CAD build for the part. Positions are in the model's coordinates, mm. Coordinates: 2 decimals unless noted, no trailing zeros. Write each loop counter-clockwise with the first axis right and the second up, starting at its lowest first coordinate (ties: lowest second). Pieces come first, ordered by that corner, then holes.
Autodesk Inventor part; units mm, degrees
ref_plane "Start Plane" through (0, 0, 0) normal (1, 0, 0) x (0, 1, 0)
ref_plane "XZ Plane" through (0, 0, 0) normal (0, 1, 0) x (-1, 0, 0)
ref_plane "XY Plane" through (0, 0, 0) normal (0, 0, 1) x (1, 0, 0)
sketch "Main Sketch" plane through (0, 0, 0) normal (0, 0, 1) x (1, 0, 0)
  line L0 (0, 0) -> (914.4, 0)
  line L1 (0, 0) -> (0, 6.35)
  line L2 (914.4, 6.35) -> (914.4, 0)
  line L3 (0, 6.35) -> (914.4, 6.35)
  dimension "d3" = 12.7
revolve "Revolution1" add sketch "Main Sketch" angle 360 about axis through (0, 0, 0) along (1, 0, 0)
chamfer "Chamfer1" distance 2.54 angle 45 1 edges at (0, -6.35, 0) measured on face at (609.6, 6.3294, -0.511)
fillet "Fillet1" radius 2.54 1 edges at (914.4, -6.35, 0)
properties part number "Shaft" material "Steel, Mild"
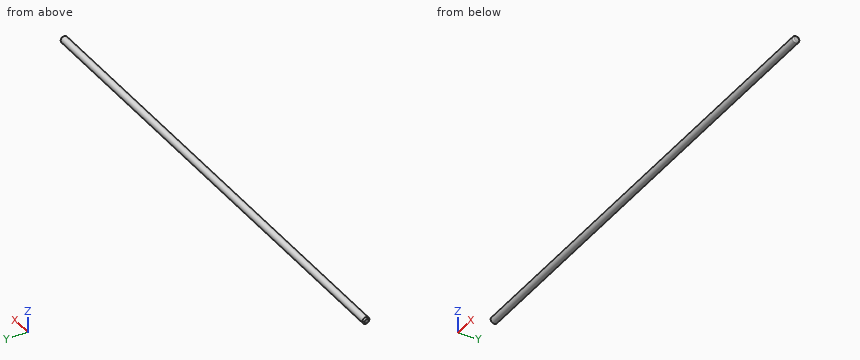
Item 1: Flat gauge pins, fed straight in: pin 1 Ø6 at (x, z) = (111.5, 3.5) entering from -Y; pin 2 Ø5 at (x, z) = (250.5, -3) entering from +Y; pin 3 Ø3 at (x, z) = (269.5, 3.5) entering from -Y. Where does each tip first touch, or does it go through?
Item 2: Saw through at A-A, the plane x = 751. Write the cut outline in (y, z).
Item 3: Wall check: line 1 along Z through (x, y) = (212, -0.75); line 2 along Z through (x, y) = (262, -5); line 3 along Y through (x, z) = (186, 0.5). Give the ranges that are in metal, low to high.
Working result:
1. pin 1: stops at y = -6.33
1. pin 2: stops at y = 6.33
1. pin 3: stops at y = -6.03
2. outline: circle Ø12.7 at (0, 0)
3. line 1: z = -6.31 to 6.31
3. line 2: z = -3.91 to 3.91
3. line 3: y = -6.33 to 6.33
